```python
from build123d import *

# Parameters (mm, degrees)
BOSS_EXTRUDE1_DEPTH = 15
SHELL1_T            = 1


with BuildPart() as part:
    # Sketch1 → Boss-Extrude1 (new body)
    with BuildSketch(Plane(origin=(0, 0, 0), x_dir=(1, 0, 0), z_dir=(0, 1, 0))):
        with BuildLine():
            ThreePointArc((25, 36.753265161), (0, 44.45), (-25, 36.753265161))
            Line((-25, 36.753265161), (-16.563554556, 24.350588504))
            ThreePointArc((-16.563554556, 24.350588504), (0, 29.45), (16.563554556, 24.350588504))
            Line((16.563554556, 24.350588504), (25, 36.753265161))
        make_face()
    extrude(amount=BOSS_EXTRUDE1_DEPTH)

    # Shell1
    shell1_openings = [part.faces().sort_by_distance(p)[0] for p in [
        (20.781777278, 7.5, -30.551926832),
        (-20.781777278, 7.5, -30.551926832),
        (0, 7.5, -29.45),
        (0, 15, -35.269418501),
    ]]
    offset(amount=SHELL1_T, openings=shell1_openings, kind=Kind.INTERSECTION)


solid = part.part
```
Could you check a few things on this model? Use its own coordinates, in mm. A direction names the side the tool comes from. Round coordinates to 2 decimals unless told otherwise and drop trailing zeros. Write each loop counter-clockwise with the first axis right and the second up, starting at its lowest first coordinate (ties: lowest second). Pieces come first, ordered by that corner, then holes. Notation, with made-up numbers: M 38.5,47.5 L 51.5,47.5 A27 ccw 51.5,71.5 Z; hole C 71.5,7 d5. An arc over 180 degrees is marked long. Write each question's results on one line, items separated by ' | '. Start each with the question number.
1. Imagine slicing it at C-C on z = -40. List the corners of the cut face in (x, y) for me.
2. Thinking about a two-plate mould opening in X: for faces 3 (the face through (0.38, 6.89, -45.45)), 4 (the face through (-0.25, -0.51, -29.45)), 5 (the face through (0, -1, -35)), 6 (the face through (23.04, -0.15, -33.87)), which applies, +X half, -X half, draft (parallel to the pull), parting line (faces both ways), or undercut?
3. On a 3-axis mill with a long thin cutter (end or side, diameter ignored), from which of +Z, -Z, +X, -X, +Y, -Y can I reach the whole of each face in a straight line? I mean faces 1 (the face through (0, 0, -35)), 2 (the face through (0, 15, -45)). Say none if no direction works.
4. I need wall thicknesses on L1, parallel to Y at x = -8.5, z = -39.25; L2, parallel to Z at x = 5.5, y = 9.5; L3, parallel to Z at x = 19, y = 1.25. Which ranges of each line are inside material? Lowest first, please. Write a range as from..to.
5. Imagine slicing it at B-B on x = 3. List the corners of the cut face in (y, z) for me.
6. Imagine slicing it at D-D on y = 12.25. List the corners of the cut face in (x, z) for me.
7. I'm going to push flat-ended pins straight in: pin 1 Ø3 at (y, z) = (6, -38) entering from +X; pin 2 Ø5 at (x, z) = (10.5, -34) entering from +Y; pin 3 Ø8 at (x, y) = (-9, 7.5) entering from -Z. Where does each tip first touch, or does it pass through?
8. Imagine slicing it at A-A on z = -25.75. List the corners of the cut face in (x, y) for me.
Result sheet:
1) outline: M -21.58,-1 L 21.58,-1 L 21.58,15 L 19.39,15 L 19.39,0 L -19.39,0 L -19.39,15 L -21.58,15 Z
2) face 3: parting line | face 4: undercut | face 5: draft | face 6: +X half
3) face 1: +Z, +Y | face 2: +Z, -Z, +X, -X, +Y
4) L1: y = -1..0 | L2: z = -45.12..-44.11 | L3: z = -41.29..-40.18
5) outline: M -1,-45.35 L 15,-45.35 L 15,-44.35 L 0,-44.35 L 0,-29.3 L -1,-29.3 Z
6) outline: M -25.56,-37.58 A45.45 ccw 25.56,-37.58 L 25,-36.75 A44.45 cw -25,-36.75 Z
7) pin 1: stops at x = 25.56 | pin 2: stops at y = 0 | pin 3: stops at z = -45.17
8) outline: M -17.52,-1 L -14.29,-1 L -14.29,0 L -17.52,0 Z; M 14.29,-1 L 17.52,-1 L 17.52,0 L 14.29,0 Z
